Source: CAD feature listing. Evaluate the final solid. Frame: model axes, mm. A direction names the side the tool comes from. Round coordinates to 2 decimals unless told otherwise and drop trailing zeros. Write each loop counter-clockwise with the first axis right and the second up, starting at its lowest first coordinate (ties: lowest second). Pieces come first, ordered by that corner, then holes.
Autodesk Inventor part; units mm, degrees
ref_plane "YZ Plane" through (0, 0, 0) normal (1, 0, 0) x (0, 1, 0)
ref_plane "XZ Plane" through (0, 0, 0) normal (0, 1, 0) x (-1, 0, 0)
ref_plane "XY Plane" through (0, 0, 0) normal (0, 0, 1) x (1, 0, 0)
sketch "Sketch1" plane through (0, 0, 0) normal (0, 1, 0) x (-1, 0, 0)
  line L0 (-59, -43) -> (59, -43)
  line L1 (59, -43) -> (59, 43)
  line L2 (59, 43) -> (-59, 43)
  line L3 (-59, 43) -> (-59, -43)
  line L4 (-59, -43) -> (59, 43) construction
  line L5 (59, -43) -> (-59, 43) construction
  line L6 (56.9723, 41.5222) -> (-57.0608, 41.5222)
  line L7 (-57.0608, 41.5222) -> (-57.0608, 34.6385)
  line L8 (-57.0608, 34.6385) -> (56.9723, 34.6385)
  line L9 (56.9723, 34.6385) -> (56.9723, 41.5222)
  line L10 (56.9723, 32.5324) -> (-57.0608, 32.5324)
  line L11 (-57.0608, 32.5324) -> (-57.0608, 25.6486)
  line L12 (-57.0608, 25.6486) -> (56.9723, 25.6486)
  line L13 (56.9723, 25.6486) -> (56.9723, 32.5324)
  line L14 (56.9723, 22.0925) -> (-57.0608, 22.0925)
  line L15 (-57.0608, 22.0925) -> (-57.0608, 15.2088)
  line L16 (-57.0608, 15.2088) -> (56.9723, 15.2088)
  line L17 (56.9723, 15.2088) -> (56.9723, 22.0925)
  line L18 (56.9723, 11.3627) -> (-57.0608, 11.3627)
  line L19 (-57.0608, 11.3627) -> (-57.0608, 4.479)
  line L20 (-57.0608, 4.479) -> (56.9723, 4.479)
  line L21 (56.9723, 4.479) -> (56.9723, 11.3627)
  line L22 (56.9723, 3.1636) -> (-57.0608, 3.1636)
  line L23 (-57.0608, 3.1636) -> (-57.0608, -3.7202)
  line L24 (-57.0608, -3.7202) -> (56.9723, -3.7202)
  line L25 (56.9723, -3.7202) -> (56.9723, 3.1636)
  line L26 (56.9723, -7.487) -> (-57.0608, -7.487)
  line L27 (-57.0608, -7.487) -> (-57.0608, -14.3707)
  line L28 (-57.0608, -14.3707) -> (56.9723, -14.3707)
  line L29 (56.9723, -14.3707) -> (56.9723, -7.487)
  line L30 (56.9723, -17.9268) -> (-57.0608, -17.9268)
  line L31 (-57.0608, -17.9268) -> (-57.0608, -24.8106)
  line L32 (-57.0608, -24.8106) -> (56.9723, -24.8106)
  line L33 (56.9723, -24.8106) -> (56.9723, -17.9268)
  line L34 (49.9475, -43) -> (-48.6509, -43)
  line L35 (-48.6509, -43) -> (-48.6509, -30.0305)
  line L36 (-48.6509, -30.0305) -> (49.9475, -30.0305)
  line L37 (49.9475, -30.0305) -> (49.9475, -43)
  point P0 (0, 0)
  dimension "d0" = 118
  dimension "d1" = 86
extrude "Extrusion1" add sketch "Sketch1" along normal blind 33 contours L3 L2 L1 L0 L37 L36 L35 | L35 L36 L37 L0 | L9 L8 L7 L6 | L13 L12 L11 L10 | L17 L16 L15 L14 | L21 L20 L19 L18 | L25 L24 L23 L22 | L29 L28 L27 L26 | L33 L32 L31 L30
sketch "Sketch2" plane through (0, 33, 0) normal (0, 1, 0) x (1, 0, 0)
  line L0 (-59, -43) -> (59, -43)
  line L1 (59, -43) -> (59, 43)
  line L2 (59, 43) -> (-59, 43)
  line L3 (-59, 43) -> (-59, -43)
  line L4 (-59, -43) -> (59, 43) construction
  line L5 (59, -43) -> (-59, 43) construction
  line L6 (56.9723, 41.5222) -> (-57.0608, 41.5222)
  line L7 (-57.0608, 41.5222) -> (-57.0608, 34.6385)
  line L8 (-57.0608, 34.6385) -> (56.9723, 34.6385)
  line L9 (56.9723, 34.6385) -> (56.9723, 41.5222)
  line L10 (56.9723, 25.6486) -> (56.9723, 32.5324)
  line L11 (-57.0608, 25.6486) -> (56.9723, 25.6486)
  line L12 (56.9723, 32.5324) -> (-57.0608, 32.5324)
  line L13 (-57.0608, 32.5324) -> (-57.0608, 25.6486)
  line L14 (56.9723, 15.2088) -> (56.9723, 22.0925)
  line L15 (-57.0608, 15.2088) -> (56.9723, 15.2088)
  line L16 (56.9723, 22.0925) -> (-57.0608, 22.0925)
  line L17 (-57.0608, 22.0925) -> (-57.0608, 15.2088)
  line L18 (56.9723, 4.479) -> (56.9723, 11.3627)
  line L19 (-57.0608, 4.479) -> (56.9723, 4.479)
  line L20 (56.9723, 11.3627) -> (-57.0608, 11.3627)
  line L21 (-57.0608, 11.3627) -> (-57.0608, 4.479)
  line L22 (56.9723, -3.7202) -> (56.9723, 3.1636)
  line L23 (-57.0608, -3.7202) -> (56.9723, -3.7202)
  line L24 (56.9723, 3.1636) -> (-57.0608, 3.1636)
  line L25 (-57.0608, 3.1636) -> (-57.0608, -3.7202)
  line L26 (56.9723, -14.3707) -> (56.9723, -7.487)
  line L27 (-57.0608, -14.3707) -> (56.9723, -14.3707)
  line L28 (56.9723, -7.487) -> (-57.0608, -7.487)
  line L29 (-57.0608, -7.487) -> (-57.0608, -14.3707)
  line L30 (56.9723, -24.8106) -> (56.9723, -17.9268)
  line L31 (-57.0608, -24.8106) -> (56.9723, -24.8106)
  line L32 (56.9723, -17.9268) -> (-57.0608, -17.9268)
  line L33 (-57.0608, -17.9268) -> (-57.0608, -24.8106)
  line L34 (49.9475, -43) -> (-48.6509, -43)
  line L35 (-48.6509, -43) -> (-48.6509, -30.0305)
  line L36 (-48.6509, -30.0305) -> (49.9475, -30.0305)
  line L37 (49.9475, -30.0305) -> (49.9475, -43)
  point P0 (0, 0)
  point P1 (0, 0)
  dimension "d4" = 118
  dimension "d5" = 86
extrude "Extrusion2" cut sketch "Sketch2" against normal blind 15 contours L35 L36 L37 L0 | L9 L8 L7 L6 | L11 L13 L12 L10 | L15 L17 L16 L14 | L19 L21 L20 L18 | L23 L25 L24 L22 | L27 L29 L28 L26 | L31 L33 L32 L30
properties part number "Motor_vez"
1) Section query C-C on z = -27.5. Return the cut outline in (x, y), then the cut area to 3 significant figures.
Taken from the geometry:
outline: (-59, 0) - (59, 0) - (59, 33) - (56.97, 33) - (56.97, 18) - (-57.06, 18) - (-57.06, 33) - (-59, 33) - close
area: 2,180 mm2
2) Contact query for flat-ended pins moving along their axis: P1, Ø2, axis at x = -14.5, z = -19.5, coming from the +Y side; P2, Ø16.5, axis at x = 2.5, y = 29, coming from the +Z side. Output: stop coordinate, or through.
Taken from the geometry:
P1: stops at y = 18
P2: stops at z = 30.03
3) Section query A-A on z = 35. Return the cut outline in (x, y), then the cut area to 3 significant figures.
Taken from the geometry:
outline: (-59, 0) - (59, 0) - (59, 33) - (49.95, 33) - (49.95, 18) - (-48.65, 18) - (-48.65, 33) - (-59, 33) - close
area: 2,420 mm2
4) Pull-direction query (Z, two-part tool) for faces 3 (the face through (56.972, 26, 11)), 4 (the face through (1, 0, 1)); classes: released by +Z, released by -Z, zero draft, split by the parting line, or undercut.
Taken from the geometry:
face 3: undercut
face 4: zero draft
5) Reachability of faces 1 (the face through (-57.061, 26, -19)), 2 (the face through (0, 18, 36)) from +Z, -Z, +X, -X, +Y, -Y: full face, straight path, thin tool, end or side. Return the list, or none.
Taken from the geometry:
face 1: +Y
face 2: +Z, +Y
6) Section query B-B on y = 21.5. State how many separate pieces and enclosed holes the cut face has, then the cut area to 3 significant figures.
Taken from the geometry:
separate pieces: 1
enclosed holes: 7
area: 3,370 mm2
7) Material intervals for line 1 (X direction, y = 21, z = 31); line 2 (Y direction, x = -16.5, z = -16); line 3 (X direction, y = 25, z = -7.5), sorted ascending.
Taken from the geometry:
line 1: x = -59 to -48.65, 49.95 to 59
line 2: y = 0 to 18
line 3: x = -59 to -57.06, 56.97 to 59
